Model file for the job. Use its own axes, mm. A direction names the side the tool comes from. Coordinates: 2 decimals unless noted, no trailing zeros. Order: outer loops, then holes, each group sorted by start corner. A loop starts at its lowest first (then second) coordinate and runs counter-clockwise, first axis right, second up.
from build123d import *

# Parameters (mm, degrees)
ESQUISSE1_W                  = 20
ESQUISSE1_H                  = 32
ESQUISSE1_R                  = 1.524
BOSS_EXTRU_1_DEPTH           = 3
BOSS_EXTRU_2_DEPTH           = 12
ENL_V_MAT_EXTRU_1_DEPTH      = 23.360679775
ENL_V_MAT_EXTRU_1_DEPTH_BACK = 23.360679775
ESQUISSE3_R                  = 2.725
ENL_V_MAT_EXTRU_2_DEPTH      = 23.360679775
ENL_V_MAT_EXTRU_2_DEPTH_BACK = 23.360679775
ESQUISSE4_R                  = 1.5
ESQUISSE5_R                  = 1.5
BOSS_EXTRU_3_DEPTH           = 1


with BuildPart() as part:
    # Esquisse1 → Boss.-Extru.1 (new body)
    with BuildSketch(Plane.XY):
        Rectangle(ESQUISSE1_W, ESQUISSE1_H)
        with Locations((0, -12.162643372)):
            Circle(ESQUISSE1_R, mode=Mode.SUBTRACT)
    extrude(amount=BOSS_EXTRU_1_DEPTH)

    # Esquisse2 → Boss.-Extru.2 (add)
    with BuildSketch(Plane.XY):
        Polygon((8, -16), (10, -16), (10, 16), (-10, 16), (-10, -16), (-8, -16), (-8, 14), (8, 14), align=None)
    extrude(amount=BOSS_EXTRU_2_DEPTH)

    # Esquisse3 → Enlèv. mat.-Extru.1 (cut, two sides: drawn at the far end of the back side and taken through both)
    with BuildSketch(Plane(origin=(0, 0, 0), x_dir=(1, 0, 0), z_dir=(0, 1, 0)).offset(-ENL_V_MAT_EXTRU_1_DEPTH_BACK)):
        with Locations(Location((0, -7.024, 0), (0, 0, 270))):
            Circle(ESQUISSE3_R)
    extrude(amount=ENL_V_MAT_EXTRU_1_DEPTH + ENL_V_MAT_EXTRU_1_DEPTH_BACK, mode=Mode.SUBTRACT)

    # Esquisse4 → Enlèv. mat.-Extru.2 (cut, two sides: drawn at the far end of the back side and taken through both)
    with BuildSketch(Plane(origin=(0, 0, 0), x_dir=(0, 0, -1), z_dir=(1, 0, 0)).offset(-ENL_V_MAT_EXTRU_2_DEPTH_BACK)):
        with Locations((-9, 9)):
            Circle(ESQUISSE4_R)
    extrude(amount=ENL_V_MAT_EXTRU_2_DEPTH + ENL_V_MAT_EXTRU_2_DEPTH_BACK, mode=Mode.SUBTRACT)

    # Esquisse5 → Boss.-Extru.3 (add)
    with BuildSketch(Plane(origin=(0, 16, 0), x_dir=(1, 0, 0), z_dir=(0, 1, 0))):
        with BuildLine():
            Line((-2, 0), (-2, 4))
            ThreePointArc((-2, 4), (0, 6), (2, 4))
            Line((2, 4), (2, 0))
            Line((2, 0), (-2, 0))
        make_face()
        with Locations(Location((0, 4, 0), (0, 0, 270))):
            Circle(ESQUISSE5_R, mode=Mode.SUBTRACT)
    extrude(amount=-BOSS_EXTRU_3_DEPTH)


solid = part.part
Q1. Cut at D-D, the plane z = 5.75. List the corners of the cut face in (x, y).
Established:
outline: (-10, -16) - (-8, -16) - (-8, 14) - (-2.41, 14) - (-2.41, 16) - (-10, 16) - close; (2.41, 14) - (8, 14) - (8, -16) - (10, -16) - (10, 16) - (2.41, 16) - close
Q2. Drop flat-ended pins along their axis: P1, Ø5, axis at x = 0, y = -12.16, coming from the -Z side; P2, Ø5, axis at y = 9, z = 9, coming from the -X side; P3, Ø2.5, axis at y = 9, z = 9, coming from the +X side; P4, Ø7, axis at x = -2.5, z = 8, coming from the -Y side. Give the stop position or say it passes through.
Established:
P1: stops at z = 0
P2: stops at x = -10
P3: passes through
P4: stops at y = 14
Q3. Cut at A-A, the plane y = 9. List the corners of the cut face in (x, z), plus the area to 3 significant figures.
Established:
outline: (-10, 0) - (10, 0) - (10, 7.5) - (8, 7.5) - (8, 3) - (-8, 3) - (-8, 7.5) - (-10, 7.5) - close; (-10, 10.5) - (-8, 10.5) - (-8, 12) - (-10, 12) - close; (8, 10.5) - (10, 10.5) - (10, 12) - (8, 12) - close
area: 84.0 mm2
Q4. Cut at B-B, the plane x = 0. List the corners of the cut face in (y, z).
Established:
outline: (-16, 0) - (-13.69, 0) - (-13.69, 3) - (-16, 3) - close; (-10.64, 0) - (15, 0) - (15, -2.5) - (16, -2.5) - (16, 4.3) - (14, 4.3) - (14, 3) - (-10.64, 3) - close; (14, 9.75) - (16, 9.75) - (16, 12) - (14, 12) - close; (15, -6) - (16, -6) - (16, -5.5) - (15, -5.5) - close
Q5. Cut at C-C, the plane z = 9. List the corners of the cut face in (x, y).
Established:
outline: (-10, -16) - (-8, -16) - (-8, 7.5) - (-10, 7.5) - close; (-10, 10.5) - (-8, 10.5) - (-8, 14) - (-1.88, 14) - (-1.88, 16) - (-10, 16) - close; (1.88, 14) - (8, 14) - (8, 10.5) - (10, 10.5) - (10, 16) - (1.88, 16) - close; (8, -16) - (10, -16) - (10, 7.5) - (8, 7.5) - close
Q6. Which spindle directions (+Z, -Z, +X, -X, +Y, -Y) get a long thin tool onto all of the face, cutting with end or side? Do faces 1 (the face through (9, 8.1, 10.2)), 2 (the face through (2, 15.5, -2)), 3 (the face through (0, 15, -2)), 4 (the face through (-8, -1, 7)), 5 (the face through (-2, 15.5, -2)). Say none if no direction does.
Established:
face 1: +X, -X
face 2: -Z, +X, +Y, -Y
face 3: -Z, +X, -X, -Y
face 4: +Z, -Y
face 5: -Z, -X, +Y, -Y
Q7. Probe line 1 (Y direction, x = -9.05, z = 9); line 2 (X direction, y = -12, z = 1.5); line 3 (X direction, y = -6.5, z = 7.5). List the from-to ranges inside material, lowest first.
Established:
line 1: y = -16 to 7.5, 10.5 to 16
line 2: x = -10 to -1.52, 1.52 to 10
line 3: x = -10 to -8, 8 to 10
Q8. Mould opens along Z. For faces 6 (the face through (0, -16, 2)), 7 (the face through (0.819, 14.986, 9.623)), 8 (the face through (0, -1, 3)) say: pulls with the +Z half, pulls with the -Z half, needs draft (parallel to the pull), parting line crosses it, or undercut.
Established:
face 6: needs draft
face 7: undercut
face 8: pulls with the +Z half
